Source: CAD feature listing. Evaluate the final solid. Frame: model axes, mm. Face numbers are marked on the shaded views. A direction names the side the tool comes from. Coordinates: 2 decimals unless noted, no trailing zeros. Order: outer loops, then holes, each group sorted by start corner. A loop starts at its lowest first (then second) coordinate and runs counter-clockwise, first axis right, second up.
```python
from build123d import *

# Parameters (mm, degrees)
F1_DEPTH = 63.5
F2_DEPTH = 25.4
F3_DEPTH = 7.9375


with BuildPart() as f1:
    # F0 (on Front) → F1 (new body, symmetric)
    with BuildSketch(Plane.XZ):
        Polygon((-41.275, 9.525), (-41.275, -9.525), (41.275, -9.525), (41.275, 9.525), (22.225, 9.525), align=None)
    extrude(amount=F1_DEPTH, both=True)

    # F0 (on Front) → F2 (join, symmetric)
    with BuildSketch(Plane.XZ):
        with BuildLine():
            Line((22.225, 9.525), (41.275, 9.525))
            Line((41.275, 9.525), (41.275, 27.0002))
            ThreePointArc((41.275, 27.0002), (45.92468, 38.22552), (57.15, 42.8752))
            Line((57.15, 42.8752), (60.325, 42.8752))
            Line((60.325, 42.8752), (60.325, 61.9252))
            Line((60.325, 61.9252), (57.15, 61.9252))
            add(Edge.make_bspline(
                [(56.099081, 61.909385), (56.450721, 61.915), (56.801044, 61.920264), (57.15, 61.9252)],
                knots=[110.543175, 110.543175, 110.543175, 110.543175, 111.504536, 111.504536, 111.504536, 111.504536], degree=3))
            ThreePointArc((56.099081, 61.909385), (32.085494, 51.321511), (22.225, 27.0002))
            Line((22.225, 27.0002), (22.225, 9.525))
        make_face()
        Polygon((111.125, 66.675), (88.400421, 66.675), (88.923447, 38.1), (111.125, 38.1), align=None)
        Polygon((60.325, 66.675), (60.325, 61.9252), (60.325, 42.8752), (60.325, 38.1), (88.923447, 38.1), (88.400421, 66.675), align=None)
    extrude(amount=F2_DEPTH, both=True)

    # F0 (on Front) → F3 (join, symmetric)
    with BuildSketch(Plane.XZ):
        with BuildLine():
            add(Edge.make_bspline(
                [(-41.275, 9.525), (-42.176598, 55.966002), (15.665411, 61.263678), (56.099081, 61.909385)],
                knots=[0, 0, 0, 0, 110.543175, 110.543175, 110.543175, 110.543175], degree=3))
            Line((-41.275, 9.525), (22.225, 9.525))
            Line((22.225, 9.525), (22.225, 27.0002))
            ThreePointArc((22.225, 27.0002), (32.085494, 51.321511), (56.099081, 61.909385))
        make_face()
    extrude(amount=F3_DEPTH, both=True)


solid = f1.part
```
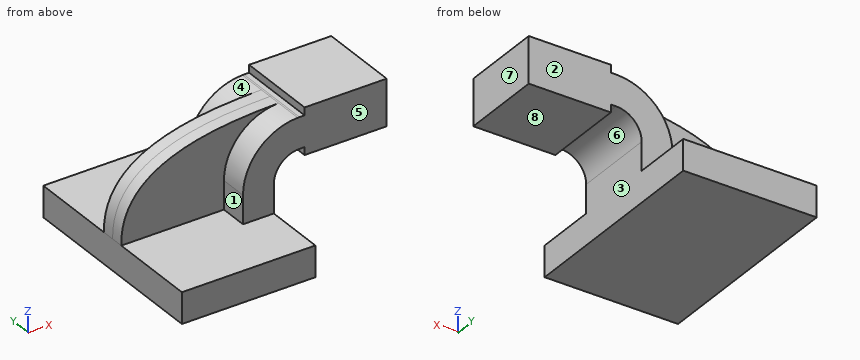
Q1. Material intervals for line 1 along X through (y, z) = (-14.5, 17) (3 decimals); line 2 along Y through (x, z) = (7.5, 53); line 3 along Z through (x, y) = (80, -8.5) (3 decimals), sorted ascending.
Solutions:
line 1: x = 22.225 to 41.275
line 2: y = -7.94 to 7.94
line 3: z = 38.1 to 66.675
Q2. Pull-direction query (X, two-part tool) for the marked faces 6, 7 and 8; classes: pulls with the +X half, pulls with the -X half, needs draft (parallel to the pull), parting line crosses it, or undercut.
Solutions:
face 6: undercut
face 7: pulls with the +X half
face 8: needs draft
Q3. Set-up query: the marked faces 1, 2, 3, 4 and 5. Return all of +Z, -Z, +X, -X, +Y, -Y with unobstructed straight access to the full face (end or side cutting, diameter ignored); none if empty.
Solutions:
face 1: +Z, -X, -Y
face 2: +Z, +X, -X, +Y
face 3: -Z, +X, +Y, -Y
face 4: +Z, -X, +Y
face 5: +Z, +X, -X, -Y
Q4. Pin query (flat end, axial travel): P1, Ø1.4, axis at y = -1.5, z = 64.5, coming from the -X side (3 decimals); P2, Ø2.5, axis at x = 59, y = -8, coming from the -Z side; P3, Ø5, axis at y = 17, z = 43, coming from the -X side. Return the tip coordinate at first contact, or that it passes through.
Solutions:
P1: stops at x = 60.325
P2: stops at z = 42.88
P3: stops at x = 24.94
Q5. Section query B-B on y = 30.5. Output: boundary loops of the cut face in (x, z) (3 decimals).
Solutions:
outline: (-41.275, -9.525) - (41.275, -9.525) - (41.275, 9.525) - (-41.275, 9.525) - close
Q6. Section query A-A on z = -3.5. Output: boundary loops of the cut face in (x, y) (3 decimals), plus the area to 3 significant figures.
Solutions:
outline: (-41.275, -63.5) - (41.275, -63.5) - (41.275, 63.5) - (-41.275, 63.5) - close
area: 10,500 mm2
